Job drawing, mm, ordinate dimensions from the low corner. One solid piece. A direction names the side the tool comes from. Round coordinates to 2 decimals unless told otherwise and drop trailing zeros. Loops run counter-clockwise (first coordinate to the right, second up) from the corner with the lowest first, then second, coordinate; pieces in that order, holes last. Notation, with made-up numbers: M 70,12.5 L 101,12.5 A27 ccw 101,47.5 Z; hole C 29.5,80 d6. An arc over 180 degrees is marked long. Use one line per item in the form item = value.
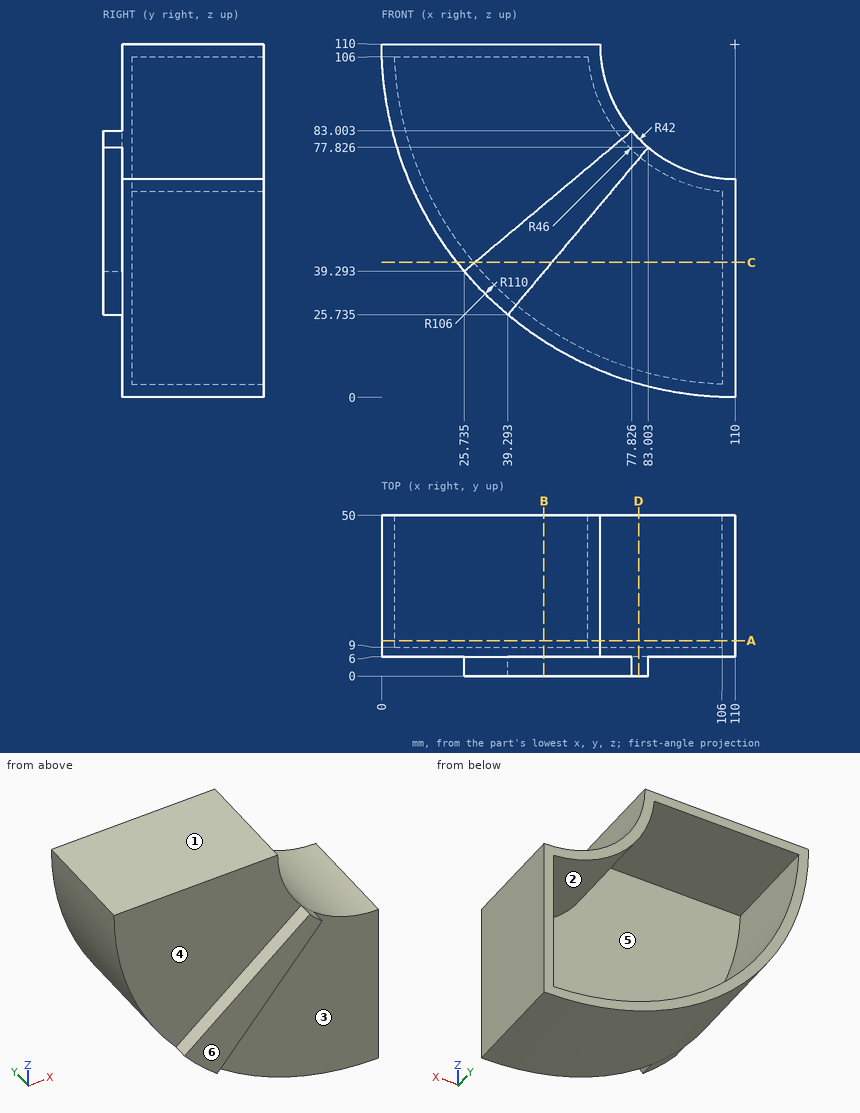
1. Probe line 1 along Y through (x, z) = (42, 33); line 2 along Y through (x, z) = (103, 58.5); line 3 along X through (y, z) = (31.5, 77.5) (1 decimal). List the from-to ranges inside material, lowest first. Write a range as from..to.
Completed:
line_1 = 0..9
line_2 = 6..9
line_3 = 4.9..9.1, 77.4..83.4
2. Tool access for the marked faces 4, 5 and 6: list every direction of +Z, -Z, +X, -X, +Y, -Y with a clear straight run to the whole face (end or side of a thin tool).
Completed:
face_4 = +Z, -X, -Y
face_5 = +Y
face_6 = +Z, -Z, +X, -X, -Y
3. Pull direction Z, two halves, no side cores. Call the marked faces 1, 2 and 3: +Z half, -Z half, draft (parallel to the pull), parting line (faces both ways), or undercut.
Completed:
face_1 = +Z half
face_2 = undercut
face_3 = draft
4. Cut at C-C on z = 42. Write the cut outline in (x, y).
Completed:
outline = M 23.54,6 L 28.96,6 L 28.96,0 L 52.94,0 L 52.94,6 L 110,6 L 110,50 L 106,50 L 106,9 L 28.69,9 L 28.69,50 L 23.54,50 Z
5. Cut at B-B on x = 50.5. Write the cut outline in (y, z) (1 decimal).
Completed:
outline = M 0,39.1 L 6,39.1 L 6,17.5 L 50,17.5 L 50,22.3 L 9,22.3 L 9,106 L 50,106 L 50,110 L 6,110 L 6,60.1 L 0,60.1 Z
6. Drop flat-ended pins along their axis: P1, Ø20.5, axis at x = 31.5, y = 30, coming from the -Z side; P2, Ø1, axis at y = 32.5, z = 70.5, coming from the -X side (1 decimal); P3, Ø6, axis at y = 11.5, z = 20.5, coming from the -X side (1 decimal). Give the stop position or say it passes through.
Completed:
P1 = 23.73
P2 = 7.1
P3 = 42
7. Cut at A-A on y = 11. Write the cut outline in (x, z) (1 decimal).
Completed:
outline = M 0,110 A110 ccw 110,0 L 110,68 A42 cw 68,110 Z; hole M 4.1,106 A106 ccw 106,4.1 L 106,64.2 A46 cw 64.2,106 Z
8. Cut at D-D on x = 80. Write the cut outline in (y, z).
Completed:
outline = M 0,74.25 L 6,74.25 L 6,4.17 L 50,4.17 L 50,8.33 L 9,8.33 L 9,75.13 L 50,75.13 L 50,80.61 L 0,80.61 Z
